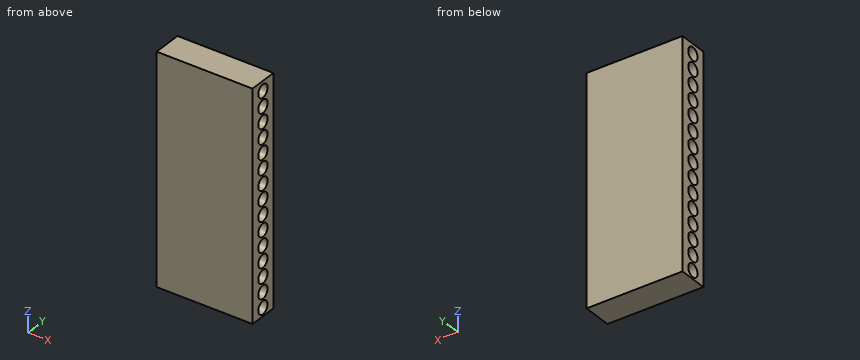
```python
from build123d import *

# Parameters (mm, degrees)
F0_W     = 14.8
F0_H     = 35
F1_DEPTH = 4.5
F2_R     = 1
F3_DEPTH = 14.801


with BuildPart() as f1:
    # F0 (on Front) → F1 (new body)
    with BuildSketch(Plane.XZ):
        Rectangle(F0_W, F0_H)
    extrude(amount=F1_DEPTH)

    # F2 (on face) → F3 (cut, through all)
    with BuildSketch(Plane(origin=(-7.4, 0, 0), x_dir=(0, -1, 0), z_dir=(-1, 0, 0))):
        with Locations((2.25, 16)):
            Circle(F2_R)
        with Locations((2.25, 13.7)):
            Circle(F2_R)
        with Locations((2.25, 11.4)):
            Circle(F2_R)
        with Locations((2.25, 9.1)):
            Circle(F2_R)
        with Locations((2.25, 6.8)):
            Circle(F2_R)
        with Locations((2.25, 4.5)):
            Circle(F2_R)
        with Locations((2.25, 2.2)):
            Circle(F2_R)
        with Locations((2.25, -0.1)):
            Circle(F2_R)
        with Locations((2.25, -2.4)):
            Circle(F2_R)
        with Locations((2.25, -4.7)):
            Circle(F2_R)
        with Locations((2.25, -7)):
            Circle(F2_R)
        with Locations((2.25, -9.3)):
            Circle(F2_R)
        with Locations((2.25, -11.6)):
            Circle(F2_R)
        with Locations((2.25, -13.9)):
            Circle(F2_R)
        with Locations((2.25, -16.2)):
            Circle(F2_R)
    extrude(amount=-F3_DEPTH, mode=Mode.SUBTRACT)


solid = f1.part
```
The listing builds one solid part. Answer for the finished solid, in the listing's coordinates (mm). Coordinates: 2 decimals unless noted, no trailing zeros. Loops run counter-clockwise (first coordinate to the right, second up) from the corner with the lowest first, then second, coordinate; pieces in that order, holes last. Notation, with made-up numbers: (-27, -17) - (-9, -17) arc R21 ccw to (-9, -6) - close; hole circle Ø5 at (87.5, 78). An arc over 180 degrees is marked (long way). Write item = value, one per line.
1) Section A-A (z = 13.7) is taken. Determine the outline of the cut face in (x, y), plus the area to 3 significant figures.
Responses:
outline = (-7.4, -4.5) - (7.4, -4.5) - (7.4, -3.25) - (-7.4, -3.25) - close; (-7.4, -1.25) - (7.4, -1.25) - (7.4, 0) - (-7.4, 0) - close
area = 37.0 mm^2
2) Find the intervals of material crossed by line 1 along Y through (x, z) = (-1, -3); line 2 along Y through (x, z) = (0.5, -12), in increasing order.
Responses:
line_1 = -4.5 to -3.05, -1.45 to 0
line_2 = -4.5 to -3.17, -1.33 to 0
3) Section B-B (x = 0) is taken. Count the separate pieces of the cut face and the enclosed holes in it, plus the area to 3 significant figures.
Responses:
separate_pieces = 1
enclosed_holes = 15
area = 110 mm^2
4) Section C-C (z = -12) is taken. Determine the outline of the cut face in (x, y).
Responses:
outline = (-7.4, -4.5) - (7.4, -4.5) - (7.4, -3.17) - (-7.4, -3.17) - close; (-7.4, -1.33) - (7.4, -1.33) - (7.4, 0) - (-7.4, 0) - close
